Source: CAD feature listing. Evaluate the final solid. Frame: model axes, mm. Face numbers are marked on the shaded views. A direction names the side the tool comes from. Give positions to 0.01 mm unless a question says otherwise; leave off trailing zeros. Order: outer loops, then holes, each group sorted by start corner. A loop starts at its lowest first (then second) coordinate and runs counter-clockwise, first axis right, second up. Notation, with made-up numbers: M -15.5,78 L -4.5,78 A25 cw -4.5,105 Z; hole C 24,-15.75 d5. An arc over 180 degrees is marked long. Answer in a Markdown table with one row per item. Add a question column.
(1) Pin query (flat end, axial travel): P1, Ø6, axis at x = 14, z = 7.5, coming from the -Y side; P2, Ø12, axis at x = 9, y = 18.5, coming from the -Z side; P3, Ø12, axis at x = -21, y = 7.5, coming from the -Z side. Return the tip coordinate at first contact, or that it passes through.
(2) Section query B-B, the plane y = 27.5. Return loops of the section in (x, z), plus the area to 3 significant figures.
(3) Section query A-A, the plane x = -39. Return loops of the section in (y, z).
(4) Material intervals for line 1 along X through (y, z) = (15.5, 10.5) (3 decimals); line 2 along Y through (x, z) = (-42.5, -18); line 3 along Y through (x, z) = (-32, -16.5), sorted ascending.
(5) Mould query, pull axis Z, two halves, no side actions, for the marked faces 3 and 4. Classes: pulls with the +Z half, pulls with the -Z half, needs draft (parallel to the pull), parting line crosses it, or undercut.
(6) Set-up query: the marked faces 1 and 2. Return all of +Z, -Z, +X, -X, +Y, -Y with unobstructed straight access to the full face (end or side cutting, diameter ignored); none if empty.
from build123d import *

# Parameters (mm, degrees)
SKETCH3_R   = 25.146
SKETCH3_R_2 = 17.526


with BuildPart() as part:
    # Sketch1 → Revolve1 (revolve)
    with BuildSketch(Plane.XY, mode=Mode.PRIVATE) as revolve1_sk:
        Polygon((-53.975, -25.146), (-22.225, -25.146), (-22.225, -21.0185), (-53.975, -21.209), align=None)
    revolve(revolve1_sk.sketch.rotate(Axis((-53.975, 0, 0), (1, 0, 0)), 270), axis=Axis((-53.975, 0, 0), (1, 0, 0)))


with BuildPart() as body_2:
    # Sketch2 → Revolve2 (revolve)
    with BuildSketch(Plane.XY, mode=Mode.PRIVATE) as revolve2_sk:
        Polygon((21.209, 53.975), (21.0185, 22.225), (25.146, 22.225), (25.146, 53.975), align=None)
    revolve(revolve2_sk.sketch.rotate(Axis((0, 0, 0), (0, 1, 0)), 90), axis=Axis((0, 0, 0), (0, 1, 0)))


with BuildPart() as sweep1_tool:
    # Sweep1: sweep along a path in Sketch4
    with BuildLine(Plane.XY) as sweep1_path:
        ThreePointArc((-22.225, 0), (-6.509552, 6.509552), (0, 22.225))
    # Sketch3 → Sweep1 (sweep)
    with BuildSketch(Plane(origin=(-22.225, 0, 0), x_dir=(0, 0, -1), z_dir=(1, 0, 0))):
        Circle(SKETCH3_R)
        Circle(SKETCH3_R_2, mode=Mode.SUBTRACT)
    sweep(path=sweep1_path.line)


with BuildPart() as part_1:
    add(part.part)


with BuildPart() as part_2:
    # Sweep1: joined with sweep1_tool
    add(part_1.part.fuse(sweep1_tool.part, body_2.part, tol=0.00001))


solid = part_2.part
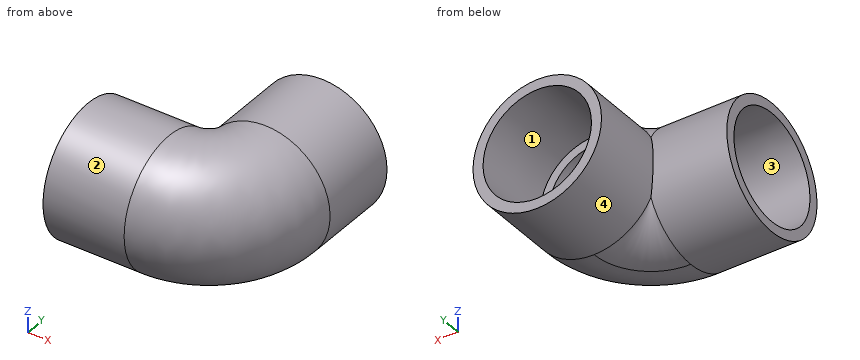
Values follow:
| question | item | result |
|---|---|---|
| 1 | P1 | stops at y = -10.16 |
| 1 | P2 | stops at z = -24.94 |
| 1 | P3 | stops at z = -25.1 |
| 2 | outline | C 0,0 d50.29; hole C 0,0 d42.1 |
| 2 | area | 594 mm² |
| 3 | outline | C 0,0 d50.29; hole C 0,0 d42.24 |
| 4 | line 1 | x = -22.225 to -17.546, 13.403 to 22.344 |
| 4 | line 2 | y = -17.56 to -11.09, 11.09 to 17.56 |
| 4 | line 3 | y = -18.98 to -13.11, 13.11 to 18.98 |
| 5 | face 3 | undercut |
| 5 | face 4 | parting line crosses it |
| 6 | face 1 | +Y |
| 6 | face 2 | -X |
